Geometry: final body of the model. Coordinates: model frame, mm. A direction names the side the tool comes from. Round coordinates to 2 decimals unless told otherwise and drop trailing zeros. Loops run counter-clockwise (first coordinate to the right, second up) from the corner with the lowest first, then second, coordinate; pieces in that order, holes last. Notation, with made-up numbers: (71.25, 0.25) - (104.25, 0.25) arc R26 ccw to (104.25, 29.25) - close; hole circle Ø10 at (-6.75, 18.25). An arc over 180 degrees is marked (long way). Return JSON: item names as keys, results as strings. Group by question number.
1. Material intervals for probe 1 along X at (y, z) = (-145, 4.5); probe 2 along X at (y, z) = (10, -85.5); probe 3 along Y at (x, z) = (-616.5, -97.5), sorted ascending.
2. Section C-C on z = -129.5. Count the separate pieces of the cut face and the enclosed holes in it, and give its area (3 significant figures).
3. Set-up query: faces 1 (the face through (543, 575, 0)), 2 (the face through (-762.4, -346.7, 0)), 3 (the face through (-458, -571.5, 7)), 4 (the face through (-768, 349, 0)). Return all of +Z, -Z, +X, -X, +Y, -Y with unobstructed straight access to the full face (end or side cutting, diameter ignored); none if empty.
4. Section D-D on x = -75. Return loops of the section in (y, z), and give its area (3 significant figures).
5. Draft query along X for faces 5 (the face through (-458, 571.5, 7)), 6 (the face through (-787.4, 3, -39)), 7 (the face through (564, -574, 0)). Return one class per face: +X half, -X half, draft (parallel to the pull), parting line (faces both ways), or undercut.
6. Section B-B on y = 108. Return loops of the section in (x, z), and give its area (3 significant figures).
7. Section A-A on x = 686. Return loops of the section in (y, z).
8. First-contact query: pin 1 Ø7.5 at (y, z) = (584, -177) entering from +X; pin 2 Ø6 at (y, z) = (-351.5, -97.5) entering from -X; pin 3 Ø2 at (x, y) = (36, -244.5) entering from -Z. Flat tips, straight axial feed; report the tip coordinate or a pass-through.
from build123d import *

# Parameters (mm, degrees)
F0_W     = 1574.8
F0_H     = 1193.8
F1_DEPTH = 25.4
F2_W     = 787.4
F2_H     = 558.8
F2_W_2   = 711.2
F2_H_2   = 330.2
F2_H_3   = 431.8
F3_DEPTH = 25.401
F4_W     = 25.4
F4_H     = 25.4
F4_H_2   = 711.2
F5_DEPTH = 292.1
F6_W     = 660.4
F6_H     = 266.7
F7_DEPTH = 50.8


with BuildPart() as f1:
    # F0 (on Top) → F1 (new body)
    with BuildSketch(Plane.XY):
        Rectangle(F0_W, F0_H)
    extrude(amount=F1_DEPTH)

    # F2 (on face) → F3 (cut, through all)
    with BuildSketch(Plane(origin=(0, 0, 0), x_dir=(1, 0, 0), z_dir=(0, 0, -1))):
        with Locations((-368.3, -292.1)):
            Rectangle(F2_W, F2_H)
        with Locations((-368.3, 292.1)):
            Rectangle(F2_W, F2_H)
        with Locations((406.4, -406.4)):
            Rectangle(F2_W_2, F2_H_2)
        with Locations((406.4, 0)):
            Rectangle(F2_W_2, F2_H_3)
        with Locations((406.4, 406.4)):
            Rectangle(F2_W_2, F2_H_2)
    extrude(amount=-F3_DEPTH, mode=Mode.SUBTRACT)

    # F4 (on face) → F5 (join)
    with BuildSketch(Plane(origin=(0, 0, 0), x_dir=(1, 0, 0), z_dir=(0, 0, -1))):
        with Locations((-622.3, 584.2)):
            Rectangle(F4_W, F4_H)
        with Locations((-622.3, -584.2)):
            Rectangle(F4_W, F4_H)
        with Locations((-774.7, 0)):
            Rectangle(F4_W, F4_H)
        with Locations((38.1, 0)):
            Rectangle(F4_W, F4_H)
        with Locations((774.7, 0)):
            Rectangle(F4_W, F4_H_2)
        with Locations((203.2, 584.2)):
            Rectangle(F4_W, F4_H)
        with Locations((203.2, -584.2)):
            Rectangle(F4_W, F4_H)
    extrude(amount=F5_DEPTH)

    # F6 (on face) → F7 (cut)
    with BuildSketch(Plane.YZ.offset(787.4)):
        with Locations((0, -133.35)):
            Rectangle(F6_W, F6_H)
    extrude(amount=-F7_DEPTH, mode=Mode.SUBTRACT)


solid = f1.part
Taken from the geometry:
{
 "1": {"probe 1": "-787.4 to -762, 25.4 to 50.8, 762 to 787.4", "probe 2": "-787.4 to -762, 25.4 to 50.8", "probe 3": "-596.9 to -571.5, 571.5 to 596.9"},
 "2": {"separate pieces": "8", "enclosed holes": "0", "area": "5,160 mm2"},
 "3": {"face 1": "-Z, +X, +Y", "face 2": "-Z, -X, -Y", "face 3": "+Z, -Z", "face 4": "-Z, -X, +Y"},
 "4": {"outline": "(-596.9, 0) - (-571.5, 0) - (-571.5, 25.4) - (-596.9, 25.4) - close; (-12.7, 0) - (12.7, 0) - (12.7, 25.4) - (-12.7, 25.4) - close; (571.5, 0) - (596.9, 0) - (596.9, 25.4) - (571.5, 25.4) - close", "area": "1,940 mm2"},
 "5": {"face 5": "undercut", "face 6": "-X half", "face 7": "draft"},
 "6": {"outline": "(-787.4, 0) - (-762, 0) - (-762, 25.4) - (-787.4, 25.4) - close; (25.4, 0) - (50.8, 0) - (50.8, 25.4) - (25.4, 25.4) - close; (762, -292.1) - (787.4, -292.1) - (787.4, -266.7) - (762, -266.7) - close; (762, 0) - (787.4, 0) - (787.4, 25.4) - (762, 25.4) - close", "area": "2,580 mm2"},
 "7": {"outline": "(-596.9, 0) - (-571.5, 0) - (-571.5, 25.4) - (-596.9, 25.4) - close; (-241.3, 0) - (-215.9, 0) - (-215.9, 25.4) - (-241.3, 25.4) - close; (215.9, 0) - (241.3, 0) - (241.3, 25.4) - (215.9, 25.4) - close; (571.5, 0) - (596.9, 0) - (596.9, 25.4) - (571.5, 25.4) - close"},
 "8": {"pin 1": "x = 215.9", "pin 2": "x = 762", "pin 3": "z = 0"}
}
